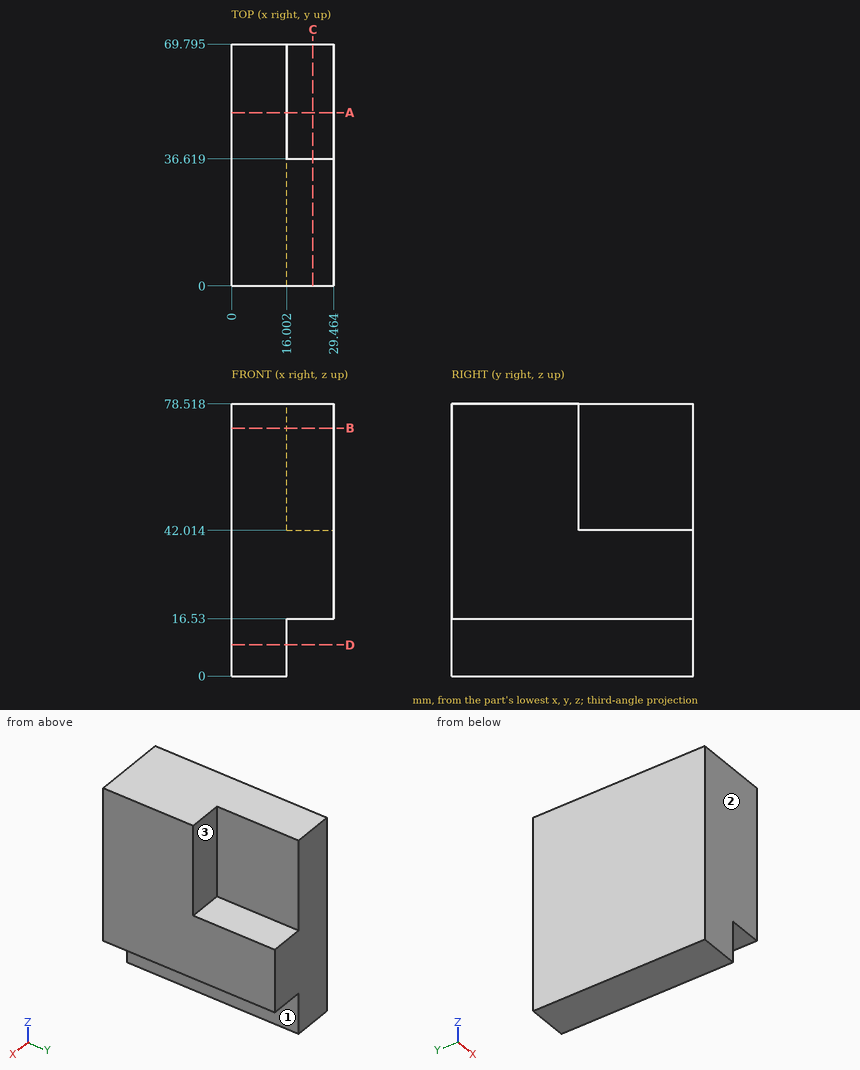
Drawing for the job (mm, zero at the part's lowest x, y, z). A direction names the side the tool comes from. Round coordinates to 2 decimals unless told otherwise and drop trailing zeros. Write each loop counter-clockwise with the first axis right and the second up, starting at its lowest first coordinate (ties: lowest second). Pieces come first, ordered by that corner, then holes. Notation, with made-up numbers: (-7.5, -20.75) - (7.5, -20.75) arc R17 ccw to (7.5, -11.75) - close; hole circle Ø10 at (0.5, -34). An arc over 180 degrees is marked (long way). Return JSON: item names as keys, results as strings. Group by question number.
Item 1: Flat gauge pins, fed straight in: pin 1 Ø6.5 at (x, y) = (24, 18.5) entering from -Z; pin 2 Ø5 at (y, z) = (32.5, 6.5) entering from +X. Where does each tip first touch, or does it go through?
Item 2: Probe probe 1 along Z at (x, y) = (28.25, 66); probe 2 along Z at (x, y) = (25.25, 35); probe 3 along X at (y, z) = (51, 7.5). List the from-to ranges inside material, lowest first.
Item 3: Band-saw the part on B-B on z = 71.5. List the corners of the cut face in (x, y) (1 decimal).
Item 4: Band-saw the part on A-A on y = 50. List the corners of the cut face in (x, z).
Item 5: 3-axis set-ups, long thin cutter, end or side, ignore diameter. For the marked faces 1, 2 and 3: which of +Z, -Z, +X, -X, +Y, -Y reach the whole face in a straight line?
Item 6: Band-saw the part on C-C on x = 23.5. List the corners of the cut face in (y, z) (1 decimal), plus the area to 3 significant figures.
Item 7: Band-saw the part on D-D on z = 9. List the corners of the cut face in (x, y) (1 decimal).
Resolved:
{
 "1": {"pin 1": "stops at z = 16.53", "pin 2": "stops at x = 16"},
 "2": {"probe 1": "z = 16.53 to 42.01", "probe 2": "z = 16.53 to 78.52", "probe 3": "x = 0 to 16"},
 "3": {"outline": "(0, 0) - (29.5, 0) - (29.5, 36.6) - (16, 36.6) - (16, 69.8) - (0, 69.8) - close"},
 "4": {"outline": "(0, 0) - (16, 0) - (16, 16.53) - (29.46, 16.53) - (29.46, 42.01) - (16, 42.01) - (16, 78.52) - (0, 78.52) - close"},
 "5": {"face 1": "-Z, +X, +Y, -Y", "face 2": "+Z, -Z, +X, -X, -Y", "face 3": "+Z, +X, +Y"},
 "6": {"outline": "(0, 16.5) - (69.8, 16.5) - (69.8, 42) - (36.6, 42) - (36.6, 78.5) - (0, 78.5) - close", "area": "3,120 mm²"},
 "7": {"outline": "(0, 0) - (16, 0) - (16, 69.8) - (0, 69.8) - close"}
}
